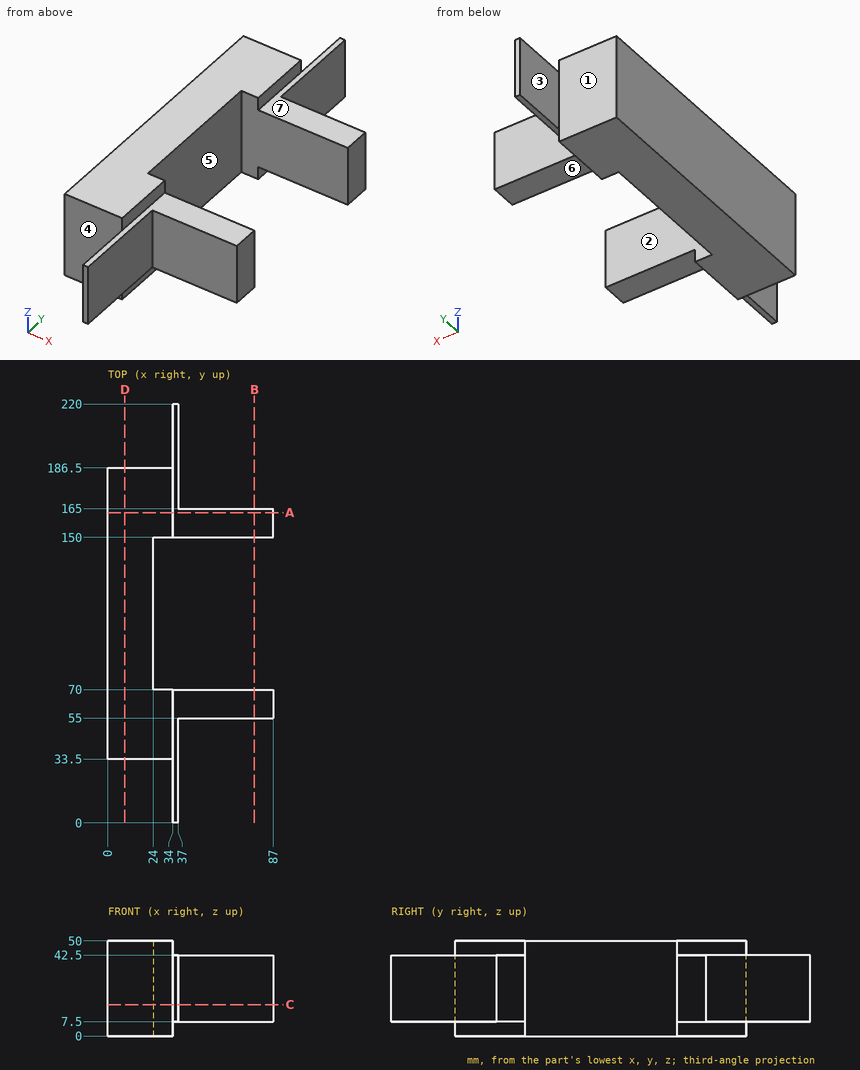
Verification items for this drawing (mm, ordinates from the low corner). A direction names the side the tool comes from. Coordinates: 2 decimals unless noted, no trailing zeros. Write each loop counter-clockwise with the first axis right and the second up, starting at its lowest first coordinate (ties: lowest second). Pieces come first, ordered by that corner, then holes. Notation, with made-up numbers: M 4.25,-26.75 L 40.25,-26.75 A23 ccw 40.25,-3.75 Z; hole C 83.5,-25.75 d11. An arc over 180 degrees is marked long. Use one line per item in the form item = value. Start each with the question number.
1) Section check C-C on z = 16.5. Enter the section's corners in (x, y), and give its area (3 significant figures).
2) Release check for a two-part mould opening along Y. For the marked faces 1, 2 and 3 record: pulls with the +Y half, pulls with the -Y half, needs draft (parallel to the pull), parting line crosses it, or undercut.
3) Section check D-D on x = 9. Enter the section's corners in (y, z), and give its area (3 significant figures).
4) Section check B-B on x = 77. Enter the section's corners in (y, z).
5) Thickness scan on probe 1 along Y at (x, z) = (80, 36.5); probe 2 along Y at (x, z) = (25, 16.5); probe 3 along Y at (x, z) = (10, 29.5). Record the ranges inside material, lowest first. Write a range as from..to.
6) Set-up check for the marked faces 4, 5, 6 and 7: record each of +Z, -Z, +X, -X, +Y, -Y from which the full face is reachable in a straight line by a thin tool's end or side.
7) Section check A-A on y = 163. Enter the section's corners in (x, z), and give its area (4 significant figures).
8) Go/stop test with flat-tipped pins: pin 1 Ø6 at (x, z) = (76, 41) entering from +Y; pin 2 Ø15 at (x, z) = (49, 18) entering from -Y; pin 3 Ø2 at (y, z) = (175, 44.5) entering from +X. Record where each tip stops, or that it passes through.
Responses:
q1.outline = M 0,33.5 L 34,33.5 L 34,0 L 37,0 L 37,55 L 87,55 L 87,70 L 24,70 L 24,150 L 87,150 L 87,165 L 37,165 L 37,220 L 34,220 L 34,186.5 L 0,186.5 Z
q1.area = 6,320 mm2
q2.face_1 = pulls with the +Y half
q2.face_2 = undercut
q2.face_3 = needs draft
q3.outline = M 33.5,0 L 186.5,0 L 186.5,50 L 33.5,50 Z
q3.area = 7,650 mm2
q4.outline = M 55,7.5 L 70,7.5 L 70,42.5 L 55,42.5 Z; M 150,7.5 L 165,7.5 L 165,42.5 L 150,42.5 Z
q5.probe_1 = 55..70, 150..165
q5.probe_2 = 33.5..70, 150..186.5
q5.probe_3 = 33.5..186.5
q6.face_4 = +Z, -Z, -X, -Y
q6.face_5 = +Z, -Z, +X
q6.face_6 = -Z, +X, +Y, -Y
q6.face_7 = +Z, +X, +Y, -Y
q7.outline = M 0,0 L 34,0 L 34,7.5 L 87,7.5 L 87,42.5 L 34,42.5 L 34,50 L 0,50 Z
q7.area = 3,555 mm2
q8.pin_1 = 165
q8.pin_2 = 55
q8.pin_3 = 34
